Here's the drawing with two shaded views (mm, measured from the low corner). I have some questions. A direction names the side the tool comes from. Round coordinates to 2 decimals unless told otherwise and drop trailing zeros. Loops run counter-clockwise (first coordinate to the right, second up) from the corner with the lowest first, then second, coordinate; pieces in that order, holes last.
(1) I want a section at A-A on x = 27.5. Write out the boundary of the cut face in (y, z) (1 decimal), plus the area to 3 significant figures.
(2) Will these pins go through, and if not, where does the flat tip stop? pin 1 Ø1 at (x, y) = (10, 11) entering from -Z; pin 2 Ø1 at (y, z) = (12.5, 3.5) entering from -X; pin 3 Ø1.5 at (x, z) = (20.5, 3.5) entering from -Y (1 decimal); pin 4 Ø1.5 at (y, z) = (37.5, 3.5) entering from -X.
(3) I want a section at B-B on y = 21.5. Write out the boundary of the cut face in (x, z), plus the area to 3 significant figures.
(4) If I drill on line 1 along X through (y, z) = (18, 3.35) (1 decimal); line 2 along Y through (x, z) = (20, 3.65) (1 decimal); line 3 along X through (y, z) = (14.5, 1.05) (1 decimal), over which ranges is the centre line in solid material (lowest first)?
(5) Which directions (+Z, -Z, +X, -X, +Y, -Y) give clear straight access to the entire face, cutting with the end or side of a thin tool? Please do the marked faces 4 and 5.
(6) Thinking about a two-plate mould opening in X: for the marked faces 1, 2 and 3, which applies, released by +X, released by -X, zero draft, split by the parting line, or undercut?
(7) I want a section at D-D on y = 16.5. Write out the boundary of the cut face in (x, z) (1 decimal), plus the area to 3 significant figures.
(8) I want a section at C-C on z = 2.8. Write out the boundary of the cut face in (x, y).
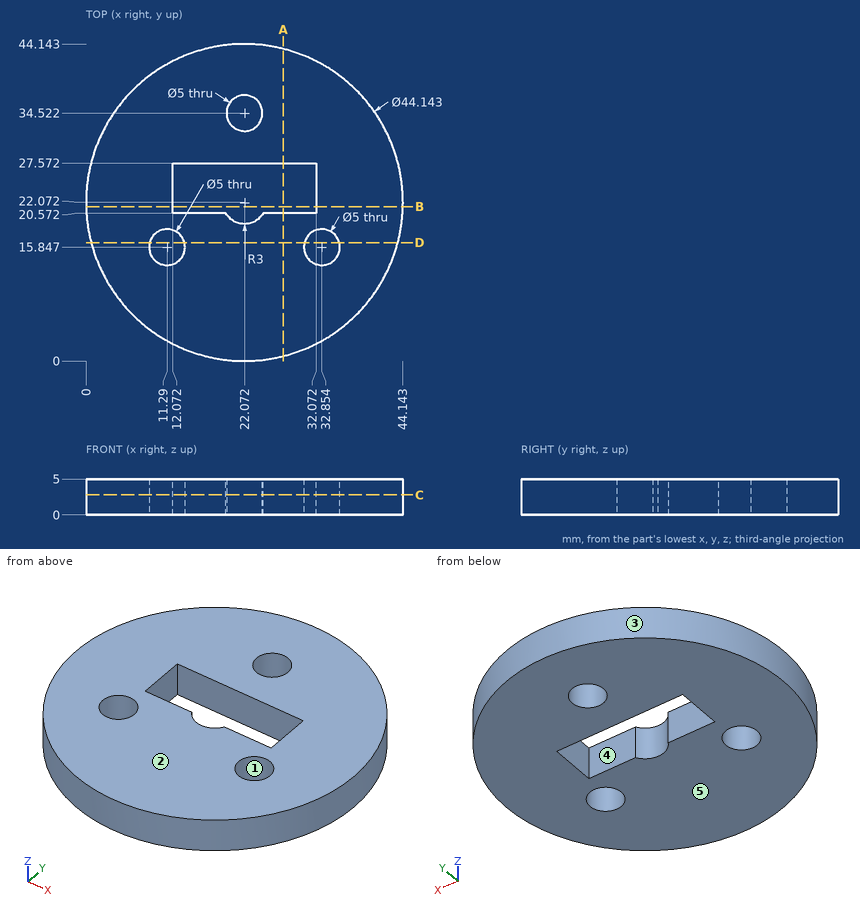
Filled sheet:
1. outline: (0.7, 0) - (20.6, 0) - (20.6, 5) - (0.7, 5) - close; (27.6, 0) - (43.5, 0) - (43.5, 5) - (27.6, 5) - close
1. area: 179 mm2
2. pin 1: stops at z = 0
2. pin 2: stops at x = 1.95
2. pin 3: stops at y = 0
2. pin 4: stops at x = 5.59
3. outline: (0.01, 0) - (12.07, 0) - (12.07, 5) - (0.01, 5) - close; (32.07, 0) - (44.14, 0) - (44.14, 5) - (32.07, 5) - close
3. area: 121 mm2
4. line 1: x = 0.4 to 10, 12.6 to 31.6, 34.1 to 43.8
4. line 2: y = 0.1 to 19.9, 27.6 to 33.1, 35.9 to 44
4. line 3: x = 1.3 to 9.2, 13.4 to 30.7, 35 to 42.8
5. face 4: +Z, -Z
5. face 5: -Z, +X, -X, +Y, -Y
6. face 1: undercut
6. face 2: zero draft
6. face 3: split by the parting line
7. outline: (0.7, 0) - (8.9, 0) - (8.9, 5) - (0.7, 5) - close; (13.7, 0) - (30.4, 0) - (30.4, 5) - (13.7, 5) - close; (35.3, 0) - (43.4, 0) - (43.4, 5) - (35.3, 5) - close
7. area: 165 mm2
8. outline: circle Ø44.14 at (22.07, 22.07); hole circle Ø5 at (11.29, 15.85); hole (12.07, 20.57) - (19.47, 20.57) arc R3 ccw to (24.67, 20.57) - (32.07, 20.57) - (32.07, 27.57) - (12.07, 27.57) - close; hole circle Ø5 at (22.07, 34.52); hole circle Ø5 at (32.85, 15.85)
